Read the model definition and answer for the solid it produces. Units are mm, in the model's axes. Face numbers are marked on the shaded views. A direction names the side the tool comes from. Coordinates: 2 decimals unless noted, no trailing zeros. Order: outer loops, then holes, each group sorted by start corner. A loop starts at its lowest first (then second) coordinate and runs counter-clockwise, first axis right, second up. Notation, with made-up numbers: M 60.25,-11.5 L 78.25,-11.5 A22 ccw 78.25,22.5 Z; hole C -15.5,6.25 d5. An arc over 180 degrees is marked long. Put each result on its own line as item: value.
from build123d import *

# Parameters (mm, degrees)
SKETCH1_W           = 25.4
SKETCH1_H           = 25.4
BOSS_EXTRUDE1_DEPTH = 25.4
SKETCH2_W           = 31.75
SKETCH2_H           = 31.75
BOSS_EXTRUDE2_DEPTH = 12.7
SKETCH3_W           = 25.4
SKETCH3_H           = 25.4
BOSS_EXTRUDE3_DEPTH = 25.4
SKETCH4_R           = 2.50825
CUT_EXTRUDE2_DEPTH  = 25.4
SKETCH5_W           = 19.05
SKETCH5_H           = 19.05
CUT_EXTRUDE3_DEPTH  = 63.5


with BuildPart() as part:
    # Sketch1 → Boss-Extrude1 (new body)
    with BuildSketch(Plane.XY):
        with Locations((-12.7, -12.7)):
            Rectangle(SKETCH1_W, SKETCH1_H)
    extrude(amount=BOSS_EXTRUDE1_DEPTH)

    # Sketch2 → Boss-Extrude2 (add)
    with BuildSketch(Plane.XY.offset(25.4)):
        with Locations((-12.7, -12.7)):
            Rectangle(SKETCH2_W, SKETCH2_H)
    extrude(amount=BOSS_EXTRUDE2_DEPTH)

    # Sketch3 → Boss-Extrude3 (add)
    with BuildSketch(Plane.XY.offset(38.1)):
        with Locations((-12.7, -12.7)):
            Rectangle(SKETCH3_W, SKETCH3_H)
    extrude(amount=BOSS_EXTRUDE3_DEPTH)

    # Sketch4 → Cut-Extrude2 (cut)
    with BuildSketch(Plane(origin=(0, 0, 0), x_dir=(0, 0, -1), z_dir=(1, 0, 0))):
        with Locations((-57.15, -6.35)):
            Circle(SKETCH4_R)
        with Locations((-44.45, -6.35)):
            Circle(SKETCH4_R)
        with Locations((-57.15, -19.05)):
            Circle(SKETCH4_R)
        with Locations((-44.45, -19.05)):
            Circle(SKETCH4_R)
    cut_extrude2 = extrude(amount=-CUT_EXTRUDE2_DEPTH, mode=Mode.SUBTRACT)

    # Sketch5 → Cut-Extrude3 (cut)
    with BuildSketch(Plane.XY.offset(63.5)):
        with Locations((-12.7, -12.7)):
            Rectangle(SKETCH5_W, SKETCH5_H)
    extrude(amount=-CUT_EXTRUDE3_DEPTH, mode=Mode.SUBTRACT)

    # Mirror1: Cut-Extrude2 across plane
    add(cut_extrude2.mirror(Plane.XY.offset(31.75)), mode=Mode.SUBTRACT)


solid = part.part
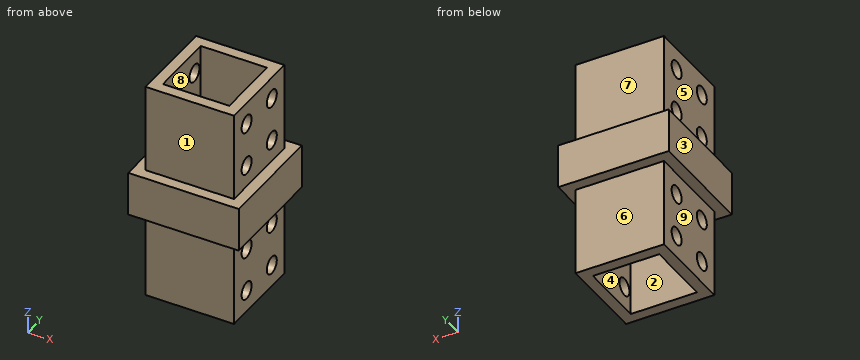
Q1. Find section A-A on z = 6.35. Write down the section's boundary in (x, y) (3 decimals), plus the area to 3 significant figures.
Answers below:
outline: M -25.4,-25.4 L 0,-25.4 L 0,-21.558 L -3.175,-21.558 L -3.175,-22.225 L -22.225,-22.225 L -22.225,-21.558 L -25.4,-21.558 Z; M -25.4,-16.542 L -22.225,-16.542 L -22.225,-8.858 L -25.4,-8.858 Z; M -25.4,-3.842 L -22.225,-3.842 L -22.225,-3.175 L -3.175,-3.175 L -3.175,-3.842 L 0,-3.842 L 0,0 L -25.4,0 Z; M -3.175,-16.542 L 0,-16.542 L 0,-8.858 L -3.175,-8.858 Z
area: 219 mm^2
Q2. A tool of negligible diameter and unlimited length cuts with its end or side. For the marked faces 5, 6, 7, 8 and 9, from which of +Z, -Z, +X, -X, +Y, -Y can it reach the whole face along a straight path? Write none if from no direction.
Answers below:
face 5: +Z, -X, +Y, -Y
face 6: -Z, +X, -X, +Y
face 7: +Z, +X, -X, +Y
face 8: +Z, -Z
face 9: -Z, -X, +Y, -Y
Q3. Find section C-C on y = -15.5. Write down the section's boundary in (x, z) (3 decimals).
Answers below:
outline: M -28.575,25.4 L -25.4,25.4 L -25.4,0 L -22.225,0 L -22.225,63.5 L -25.4,63.5 L -25.4,38.1 L -28.575,38.1 Z; M -3.175,0 L 0,0 L 0,25.4 L 3.175,25.4 L 3.175,38.1 L 0,38.1 L 0,63.5 L -3.175,63.5 Z
Q4. For a pull along X with two mould halves and no side action, classify the marked faces 1, 2, 3 and 4 as +X half, -X half, draft (parallel to the pull), parting line (faces both ways), or undercut.
Answers below:
face 1: draft
face 2: undercut
face 3: -X half
face 4: undercut
Q5. Find section B-B on x = -2. Give the number of separate pieces and of enclosed holes in the cut face, plus the area to 3 significant figures.
Answers below:
separate pieces: 1
enclosed holes: 8
area: 1,540 mm^2
Q6. Consider line 1 along Y through (x, z) = (-23.35, 6.35); line 2 along Y through (x, z) = (-23, 44); line 3 along Y through (x, z) = (-10, 23) (3 decimals). Determine where each line is inside the solid, lowest interval first.
Answers below:
line 1: y = -25.4 to -21.56, -16.54 to -8.86, -3.84 to 0
line 2: y = -25.4 to -21.52, -16.58 to -8.82, -3.88 to 0
line 3: y = -25.4 to -22.225, -3.175 to 0
Q7. Find section D-D on y = -23. Write down the section's boundary in (x, z) (3 decimals).
Answers below:
outline: M -28.575,25.4 L -25.4,25.4 L -25.4,0 L 0,0 L 0,25.4 L 3.175,25.4 L 3.175,38.1 L 0,38.1 L 0,63.5 L -25.4,63.5 L -25.4,38.1 L -28.575,38.1 Z
Q8. Given pin 1 (1 mm diameter, centred on x = -15.5, z = 54.5, fed in from -Y); pin 2 (9.5 mm diameter, centred on x = -10.5, y = -11.5, fed in from +Z); pin 3 (2 mm diameter, centred on y = -1, z = 55.5, fed in from +X); pin 4 (2 mm diameter, centred on y = -19.5, z = 40.5, fed in from -X), each flat-ended and moving along its own axis, determine where each tip first touches the part or whether it passes through.
Answers below:
pin 1: stops at y = -25.4
pin 2: passes through
pin 3: stops at x = 0
pin 4: stops at x = -25.4
